Read the model definition and answer for the solid it produces. Units are mm, in the model's axes. Face numbers are marked on the shaded views. A direction names the side the tool comes from. Give positions to 0.01 mm unless a question says otherwise; leave off trailing zeros. Order: outer loops, then holes, each group sorted by start corner. A loop starts at its lowest first (then second) coordinate and runs counter-clockwise, first axis right, second up.
Item 1: A cutting plane is placed at A-A (y = 0). Write down the section's boundary in (x, z), plus the area to 4 significant figures.
Item 2: Find the intervals of material crossed by line 1 along Y through (x, z) = (7, 5); line 2 along Y through (x, z) = (9.25, 0); line 3 along Y through (x, z) = (6, 0.25), in increasing order.
Item 3: Given pin 1 Ø4 at (x, z) = (28, 4.5) entering from -Y; pin 2 Ø3.5 at (y, z) = (0, 1) entering from +X; pin 3 Ø2.5 at (y, z) = (-9, -0.5) entering from +X, each flat-ended and moving along its own axis, determine where each tip first touches the part or whether it passes through.
Item 4: A cutting plane is placed at C-C (y = -6). Write down the section's boundary in (x, z).
Item 5: The mould has two halves that part along Z. Classify the marked faces 1, 2, 3 and 4: +Z half, -Z half, draft (parallel to the pull), parting line (faces both ways), or undercut.
Item 6: A cutting plane is placed at D-D (z = -0.5). Write down the section's boundary in (x, y), plus the area to 3 significant figures.
Item 7: Which of the six approach directions +Z, -Z, +X, -X, +Y, -Y give full straight-line access (tool end or side, diameter ignored) to the marked faces 5, 6, 7 and 8?
Item 8: A cutting plane is placed at B-B (z = 1.25). Write down the section's boundary in (x, y).
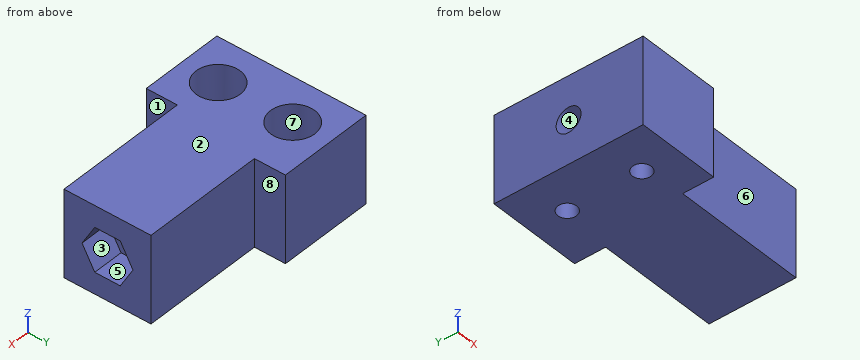
from build123d import *

# Parameters (mm, degrees)
ESQUISSE1_W             = 14
ESQUISSE1_H             = 14
BOSS_EXTRU_1_DEPTH      = 35
ESQUISSE2_R             = 2
ENL_V_MAT_EXTRU_1_DEPTH = 37.373066959
ENL_V_MAT_EXTRU_2_DEPTH = 5
ESQUISSE4_W             = 15.325652572
ESQUISSE4_H             = 14
BOSS_EXTRU_2_DEPTH      = 5
ESQUISSE5_W             = 13.435346111
ESQUISSE5_H             = 14
BOSS_EXTRU_3_DEPTH      = 5
ESQUISSE6_R             = 1.5
ENL_V_MAT_EXTRU_3_DEPTH = 40.56008089
ESQUISSE7_R             = 3.55
ENL_V_MAT_EXTRU_4_DEPTH = 8


with BuildPart() as part:
    # Esquisse1 → Boss.-Extru.1 (new body)
    with BuildSketch(Plane(origin=(0, 0, 0), x_dir=(0, 0, -1), z_dir=(1, 0, 0))):
        Rectangle(ESQUISSE1_W, ESQUISSE1_H)
    extrude(amount=BOSS_EXTRU_1_DEPTH)

    # Esquisse2 → Enlèv. mat.-Extru.1 (cut, through all)
    with BuildSketch(Plane.ZY):
        Circle(ESQUISSE2_R)
    extrude(amount=-ENL_V_MAT_EXTRU_1_DEPTH, mode=Mode.SUBTRACT)

    # Esquisse3 → Enlèv. mat.-Extru.2 (cut)
    with BuildSketch(Plane(origin=(35, 0, 0), x_dir=(0, 0, -1), z_dir=(1, 0, 0))):
        Polygon((3.55, -2.049593456), (3.55, 2.049593456), (0, 4.099186911), (-3.55, 2.049593456), (-3.55, -2.049593456), (0, -4.099186911), align=None)
    extrude(amount=-ENL_V_MAT_EXTRU_2_DEPTH, mode=Mode.SUBTRACT)

    # Esquisse4 → Boss.-Extru.2 (add)
    with BuildSketch(Plane(origin=(0, 7, 0), x_dir=(1, 0, 0), z_dir=(0, 1, 0))):
        with Locations((7.662826286, 0)):
            Rectangle(ESQUISSE4_W, ESQUISSE4_H)
    extrude(amount=BOSS_EXTRU_2_DEPTH)

    # Esquisse5 → Boss.-Extru.3 (add)
    with BuildSketch(Plane.XZ.offset(7)):
        with Locations((6.717673056, 0)):
            Rectangle(ESQUISSE5_W, ESQUISSE5_H)
    extrude(amount=BOSS_EXTRU_3_DEPTH)

    # Esquisse6 → Enlèv. mat.-Extru.3 (cut, through all)
    with BuildSketch(Plane.XY.offset(7)):
        with Locations((6.850460042, 6)):
            Circle(ESQUISSE6_R)
        with Locations((6.850460042, -6)):
            Circle(ESQUISSE6_R)
    extrude(amount=-ENL_V_MAT_EXTRU_3_DEPTH, mode=Mode.SUBTRACT)

    # Esquisse7 → Enlèv. mat.-Extru.4 (cut)
    with BuildSketch(Plane.XY.offset(7)):
        with Locations((6.850460042, 6)):
            Circle(ESQUISSE7_R)
        with Locations((6.850460042, -6)):
            Circle(ESQUISSE7_R)
    extrude(amount=-ENL_V_MAT_EXTRU_4_DEPTH, mode=Mode.SUBTRACT)


solid = part.part
Response values:
1. outline: (0, -7) - (35, -7) - (35, -3.55) - (30, -3.55) - (30, -2) - (0, -2) - close; (0, 2) - (30, 2) - (30, 3.55) - (35, 3.55) - (35, 7) - (0, 7) - close
1. area: 334.5 mm2
2. line 1: y = -12 to -9.55, -2.45 to 2.45, 9.55 to 12
2. line 2: y = -12 to -8.62, -3.38 to -2, 2 to 3.38, 8.62 to 12
2. line 3: y = -12 to -9.45, -2.55 to -1.98, 1.98 to 2.55, 9.45 to 12
3. pin 1: stops at y = -7
3. pin 2: stops at x = 30
3. pin 3: stops at x = 13.44
4. outline: (0, -7) - (5.35, -7) - (5.35, -1) - (3.3, -1) - (3.3, 7) - (0, 7) - close; (8.35, -7) - (35, -7) - (35, 7) - (10.4, 7) - (10.4, -1) - (8.35, -1) - close
5. face 1: draft
5. face 2: +Z half
5. face 3: undercut
5. face 4: undercut
6. outline: (0, -12) - (13.44, -12) - (13.44, -7) - (35, -7) - (35, -3.81) - (30, -3.81) - (30, -1.94) - (0, -1.94) - close; (0, 1.94) - (30, 1.94) - (30, 3.81) - (35, 3.81) - (35, 7) - (15.33, 7) - (15.33, 12) - (0, 12) - close; hole circle Ø7.1 at (6.85, -6); hole circle Ø7.1 at (6.85, 6)
6. area: 400 mm2
7. face 5: +X
7. face 6: +Z, -Z, +X, -Y
7. face 7: +Z
7. face 8: +Z, -Z, +X, +Y
8. outline: (0, -12) - (13.44, -12) - (13.44, -7) - (35, -7) - (35, -3.38) - (30, -3.38) - (30, -1.56) - (0, -1.56) - close; (0, 1.56) - (30, 1.56) - (30, 3.38) - (35, 3.38) - (35, 7) - (15.33, 7) - (15.33, 12) - (0, 12) - close; hole circle Ø7.1 at (6.85, -6); hole circle Ø7.1 at (6.85, 6)
